from build123d import *

# Parameters (mm, degrees)
BOSS_EXTRUDE1_DEPTH = 3.81
FILLET1_R           = 2.54


with BuildPart() as part:
    # Sketch2 → Boss-Extrude1 (new body)
    with BuildSketch(Plane.XY):
        Polygon((-24.165117367, -826.289827771), (140.930897986, -980.294891713), (140.930897986, -1065.870274418), (-36.694836072, -980.294891713), (-36.694836072, -826.289827771), align=None)
    extrude(amount=BOSS_EXTRUDE1_DEPTH)

    # Fillet1
    # the kernel refuses this fillet: 2.54 mm, written as the material it takes off along each edge
    with BuildSketch(Plane(origin=(-28.808504328, -821.958377953, 3.81), x_dir=(0, 0, -1), z_dir=(0.7312420410589273, -0.6821180817043146, 0))) as fillet1_piece_1:
        with BuildLine():
            CenterArc((FILLET1_R, -FILLET1_R), FILLET1_R, 90, 90)
            Line((0, -FILLET1_R), (0, 0))
            Line((0, 0), (FILLET1_R, 0))
        make_face()
    extrude(amount=238.474786026, mode=Mode.SUBTRACT)
    with BuildSketch(Plane(origin=(-28.808504328, -821.958377953, 0), x_dir=(0, 0, 1), z_dir=(0.7312420410589273, -0.6821180817043146, 0))) as fillet1_piece_2:
        with BuildLine():
            CenterArc((FILLET1_R, FILLET1_R), FILLET1_R, 180, 90)
            Line((0, FILLET1_R), (0, 0))
            Line((0, 0), (FILLET1_R, 0))
        make_face()
    extrude(amount=238.474786026, mode=Mode.SUBTRACT)


solid = part.part
Can you work these out from the model? Positions are in its coordinate system, mm. Give positions to 0.01 mm unless a question says otherwise; leave off trailing zeros. Loops run counter-clockwise (first coordinate to the right, second up) from the corner with the lowest first, then second, coordinate; pieces in that order, holes last. Notation, with made-up numbers: (5.25, 41) - (30.25, 41) arc R8 cw to (30.25, 46) - close; hole circle Ø11 at (56, 17.25). An arc over 180 degrees is marked (long way). Return JSON: item names as keys, results as strings.
1. If I drill on line 1 (X direction, y = -1031, z = 2.55); line 2 (X direction, y = -934.5, z = 3.1); line 3 (Y direction, x = 98.5, z = 0.7), over which ranges is the centre line in solid material (lowest first)?
Output values:
{"line 1": "x = 68.55 to 140.93", "line 2": "x = -36.69 to 90.7", "line 3": "y = -1045.43 to -941.79"}
2. I'm going to push a flat-ended pin straight in: pin 1 Ø8 at (x, y) = (58, -1025.5) entering from -Z. Where does the tip first touch, or does it pass through?
Output values:
{"pin 1": "stops at z = 0"}
3. I want a section at A-A on z = 2.75. Please give me the cut outline in (x, y).
Output values:
{"outline": "(-36.69, -980.29) - (140.93, -1065.87) - (140.93, -980.95) - (-24.86, -826.29) - (-36.69, -826.29) - close"}
4. I want a section at B-B on y = -1022. Please give me the cut outline in (x, z).
Output values:
{"outline": "(49.87, 0) - (140.93, 0) - (140.93, 3.81) - (49.87, 3.81) - close"}
